Build history of the part. All positions in model axes, mm. A direction names the side the tool comes from. Round coordinates to 2 decimals unless told otherwise and drop trailing zeros. Write each loop counter-clockwise with the first axis right and the second up, starting at its lowest first coordinate (ties: lowest second). Pieces come first, ordered by that corner, then holes. Notation, with made-up numbers: M 11.25,54 L 23.25,54 A16 ccw 23.25,81 Z; hole C -5,31 d3. An arc over 180 degrees is marked long. Write item = value, one per line.
Autodesk Inventor part; units mm, degrees
ref_plane "YZ Plane" through (0, 0, 0) normal (1, 0, 0) x (0, 1, 0)
ref_plane "XZ Plane" through (0, 0, 0) normal (0, 1, 0) x (-1, 0, 0)
ref_plane "XY Plane" through (0, 0, 0) normal (0, 0, 1) x (1, 0, 0)
sketch "Sketch1" plane through (0, 0, 0) normal (0, 1, 0) x (-1, 0, 0)
  circle A0 centre (0, 0) radius 20
  dimension "d0" = 40
extrude "Extrusion1" add sketch "Sketch1" along normal blind 6
sketch "Sketch3" plane through (0, 6, 0) normal (0, 1, 0) x (1, 0, 0)
  line L0 (0, 0) -> (0, 20)
  circle A0 centre (0, 0) radius 20
  line L1 (5, 35) -> (5, 5)
  line L2 (5, 5) -> (-5, 5)
  line L3 (-5, 5) -> (-5, 35)
  line L4 (-5, 35) -> (5, 35)
  line L5 (5, 35) -> (-5, 5) construction
  line L6 (5, 5) -> (-5, 35) construction
  line L7 (20, 0) -> (-20, 0) construction
  line L8 (5, -35) -> (5, -5)
  line L9 (5, -5) -> (-5, -5)
  line L10 (-5, -5) -> (-5, -35)
  line L11 (-5, -35) -> (5, -35)
  point P0 (-5, 19.3649)
  point P1 (5, 19.3649)
  point P2 (-5, -19.3649)
  point P3 (5, -19.3649)
  dimension "d11" = 30
  dimension "d12" = 10
extrude "Extrusion2" cut sketch "Sketch3" against normal blind 2 contours L2 L3 A0 L0 | L0 A0 L1 L2 | L10 L9 L8 A0
sketch "Sketch5" plane through (0, 4, 0) normal (0, 1, 0) x (1, 0, 0)
  circle A0 centre (0, -8) radius 1
  circle A1 centre (0, -15) radius 1
  line L0 (-5, -5) -> (5, -5)
  arc A2 (-5, 19.3649) -> (-5, -19.3649) centre (0, 0) ccw
  line L1 (-20, 0) -> (20, 0) construction
  arc A3 (5, -19.3649) -> (5, 19.3649) centre (0, 0) ccw
  circle A4 centre (0, 8) radius 1
  circle A5 centre (0, 15) radius 1
  line L2 (5, 5) -> (-5, 5)
  line L3 (5, 19.3649) -> (5, 5)
  dimension "d20" = 2
  dimension "d21" = 2
  dimension "d22" = 3
  dimension "d23" = 7
  dimension "d39" = 3
  dimension "d40" = 5
  dimension "d41" = 5
hole "Hole2" at (0, 4, 15) at (0, 4, 8) at (0, 4, -8) at (0, 4, -15) direction (0, -1, 0) diameter 3.4 depth 10.979 tip angle 118
sketch "Sketch6" plane through (0, 0, 0) normal (0, -1, 0) x (1, 0, 0)
  circle A0 centre (0, 0) radius 1.5
  dimension "d31" = 3
hole "Hole3" at (0, 0, 0) direction (0, 1, 0) diameter 5.5 depth 8.8 tip angle 118 countersink diameter 6.8 countersink angle 90
properties part number "prop_retaining_part"
1. Tool access for faces 4 (the face through (0, 5, 5)), 5 (the face through (5, 5, -12)), 6 (the face through (-0.51, 1.97, -13.38)): list every direction of +Z, -Z, +X, -X, +Y, -Y with a clear straight run to the whole face (end or side of a thin tool).
Responses:
face_4 = +Z, +Y
face_5 = -Z, +Y
face_6 = +Y, -Y
2. Flat gauge pins, fed straight in: pin 1 (1.5 mm diameter, centred on y = 3.5, z = 8, fed in from +X); pin 2 (5 mm diameter, centred on x = 0, z = 0, fed in from +Y); pin 3 (11 mm diameter, centred on x = -2, z = -13, fed in from +Y); pin 4 (1.5 mm diameter, centred on y = 2.5, z = 12, fed in from +X). Where does each tip first touch, or does it go through?
Responses:
pin_1 = 18.64
pin_2 = through
pin_3 = 6
pin_4 = 16.54
3. Mould opens along X. For faces 1 (the face through (-4, 6, 0)), 2 (the face through (1.03, 1.97, 6.65)), 3 (the face through (-18.475, 2.958, 7.66)) say: pulls with the +X half, pulls with the -X half, needs draft (parallel to the pull), parting line crosses it, or undercut.
Responses:
face_1 = needs draft
face_2 = undercut
face_3 = parting line crosses it
4. Probe probe 1 along Z at (x, y) = (0, 2.6); probe 2 along Z at (x, y) = (0, 4.8); probe 3 along Y at (x, z) = (3.5, 6.5). List the from-to ranges inside material, lowest first.
Responses:
probe_1 = -20 to -16.7, -13.3 to -9.7, -6.3 to -2.75, 2.75 to 6.3, 9.7 to 13.3, 16.7 to 20
probe_2 = -5 to -2.75, 2.75 to 5
probe_3 = 0 to 4
5. Band-saw the part on D-D (y = 2). List the corners of the cut face in (x, z).
Responses:
outline = C 0,0 d40; hole C 0,0 d5.5; hole C 0,-15 d3.4; hole C 0,-8 d3.4; hole C 0,8 d3.4; hole C 0,15 d3.4
6. Band-saw the part on A-A (x = 0). Count the separate pieces of the cut face and the enclosed holes in it, plus the area to 3 significant figures.
Responses:
separate_pieces = 6
enclosed_holes = 0
area = 92.2 mm²
7. Band-saw the part on B-B (y = 5.15). List the corners of the cut face in (x, z).
Responses:
outline = M -5,-19.36 L -5,-5 L 5,-5 L 5,-19.36 A20 ccw 5,19.36 L 5,5 L -5,5 L -5,19.36 A20 ccw Z; hole C 0,0 d5.5
8. Band-saw the part on C-C (z = -14). List the corners of the cut face in (x, y).
Responses:
outline = M -14.28,0 L -1.37,0 L -1.37,4 L -5,4 L -5,6 L -14.28,6 Z; M 1.37,0 L 14.28,0 L 14.28,6 L 5,6 L 5,4 L 1.37,4 Z
